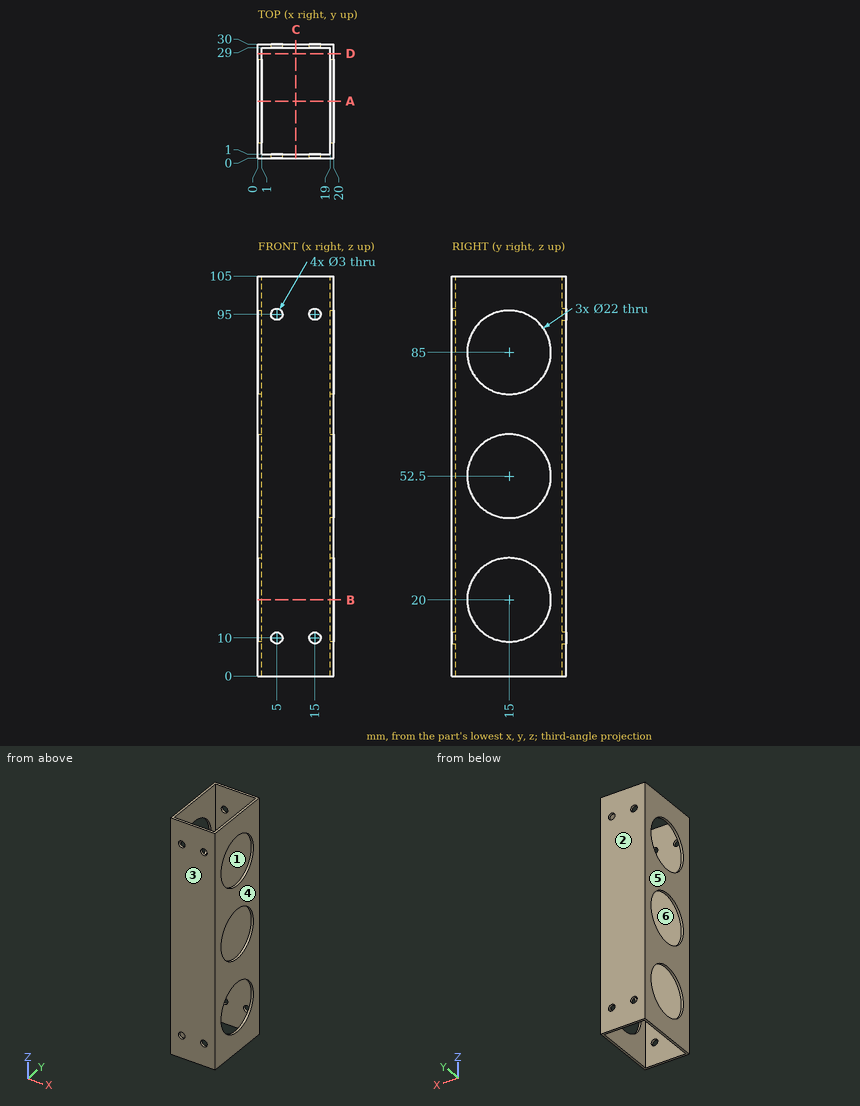
Check sheet for the drawn part. Datum: minimum x, y, z corner. Units: mm. A direction names the side the tool comes from. Round coordinates to 2 decimals unless told otherwise and drop trailing zeros. Loops run counter-clockwise (first coordinate to the right, second up) from the corner with the lowest first, then second, coordinate; pieces in that order, holes last. Notation, with made-up numbers: (-20, -31.75) - (28, -31.75) arc R15 cw to (28, -7.75) - close; hole circle Ø1 at (37, -30). An arc over 180 degrees is marked (long way). Answer as a JSON object with one key per item and string values. Group by question number.
Q1. Sectioned sample at C-C, the plane x = 10. Enter the section's corners in (y, z), plus the area to 3 significant figures.
Q2. Sectioned sample at B-B, the plane z = 20. Enter the section's corners in (x, y), plus the area to 3 significant figures.
Q3. Sectioned sample at D-D, the plane y = 27.5. Enter the section's corners in (x, z).
Q4. Gauge pin test, flat end, axial feed: P1, Ø17.5, axis at y = 15, z = 52.5, coming from the +X side. Record the tip position at first contact, or that the pin passes through.
Q5. Scan lines: line 1 along X through (y, z) = (29.8, 95); line 2 along X through (y, z) = (16, 5.5); line 3 along Y through (x, z) = (8, 7.5). Record each from-to range of solid material in increasing order. Write a range as [from, to].
Q6. Mould release check, pull along Y, two halves, no side actions. Record for the marked faces 1, 2, 3 and 4: released by +Y, released by -Y, zero draft, split by the parting line, or undercut.
Q7. Sectioned sample at A-A, the plane y = 15. Count the separate pieces of the cut face and the enclosed holes in it, plus the area to 3 significant figures.
Q8. Set-up check for the marked faces 5 and 6: record each of +Z, -Z, +X, -X, +Y, -Y from which the full face is reachable in a straight line by a thin tool's end or side.
Solution:
{
 "1": {"outline": "(0, 0) - (1, 0) - (1, 105) - (0, 105) - close; (29, 0) - (30, 0) - (30, 105) - (29, 105) - close", "area": "210 mm²"},
 "2": {"outline": "(0, 0) - (20, 0) - (20, 4) - (19, 4) - (19, 1) - (1, 1) - (1, 4) - (0, 4) - close; (0, 26) - (1, 26) - (1, 29) - (19, 29) - (19, 26) - (20, 26) - (20, 30) - (0, 30) - close", "area": "52.0 mm²"},
 "3": {"outline": "(0, 0) - (1, 0) - (1, 105) - (0, 105) - close; (19, 0) - (20, 0) - (20, 105) - (19, 105) - close"},
 "4": {"P1": "passes through"},
 "5": {"line 1": "x = [0, 3.5], [6.5, 13.5], [16.5, 20]", "line 2": "x = [0, 1], [19, 20]", "line 3": "y = [0, 1], [29, 30]"},
 "6": {"face 1": "undercut", "face 2": "released by +Y", "face 3": "released by -Y", "face 4": "zero draft"},
 "7": {"separate pieces": "8", "enclosed holes": "0", "area": "78.0 mm²"},
 "8": {"face 5": "+Z, -Z, -X, +Y, -Y", "face 6": "+Z, -Z"}
}
